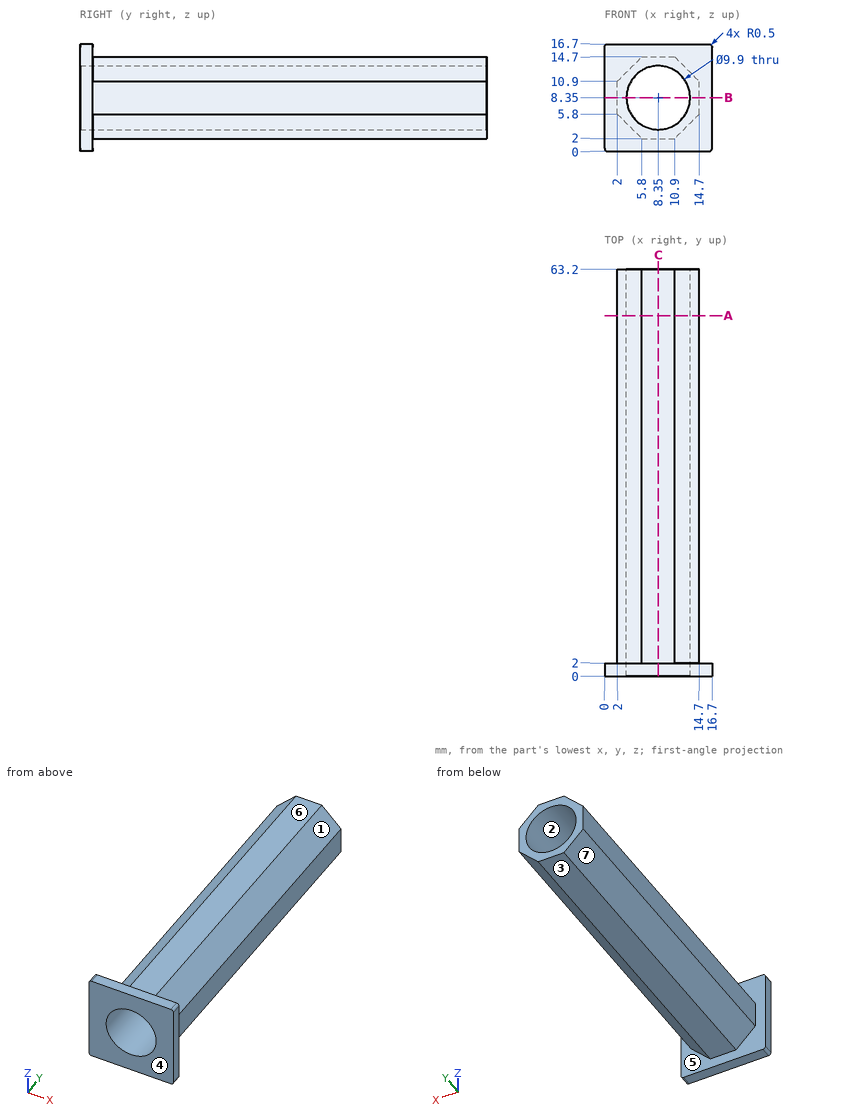
Verification items for this drawing (mm, ordinates from the low corner). A direction names the side the tool comes from. Coordinates: 2 decimals unless noted, no trailing zeros. Loops run counter-clockwise (first coordinate to the right, second up) from the corner with the lowest first, then second, coordinate; pieces in that order, holes last. Notation, with made-up numbers: (82, 11.5) - (108, 11.5) arc R20 cw to (108, 41.5) - close; hole circle Ø10 at (-20, 54.5). An arc over 180 degrees is marked (long way). One line per item, written item: value. Start each with the question number.
(1) Tool access check on the marked faces 4, 5, 6 and 7. Record the directions out of +Z, -Z, +X, -X, +Y, -Y that give a thin tool (end or side, any length) a straight path to the whole face; none if there is none.
(2) Mould release check, pull along X, two halves, no side actions. Record for the marked faces 1, 2 and 3: released by +X, released by -X, zero draft, split by the parting line, or undercut.
(3) Cross-section at C-C on x = 8.35. Enter the section's corners in (y, z), plus the area to 3 significant figures.
(4) Depth check by flat-ended pin: P1, Ø5.5, axis at x = 8, y = 34, coming from the +Z side; P2, Ø3, axis at x = 12.5, y = 12, coming from the -Z side; P3, Ø1.5, axis at y = 31, z = 9, coming from the -X side. Enter the tip coordinate at first touch or a pass-through.
(5) Cross-section at A-A on y = 56. Enter the section's corners in (x, z).
(6) Cross-section at B-B on z = 8.35. Enter the section's corners in (x, y).
(7) Material ranges on line 1 (Z direction, x = 8.35, y = 30); line 2 (Y direction, x = 3.5, z = 1.5); line 3 (Z direction, x = 10.25, y = 38), recorded low to high. Write a range as [from, to].
Results below:
1. face 4: +Z, -Z, +X, -X, -Y
1. face 5: +Y
1. face 6: +Z, +X, -X, +Y
1. face 7: -Z, -X, +Y
2. face 1: released by +X
2. face 2: undercut
2. face 3: zero draft
3. outline: (0, 0) - (2, 0) - (2, 2) - (63.2, 2) - (63.2, 3.4) - (0, 3.4) - close; (0, 13.3) - (63.2, 13.3) - (63.2, 14.7) - (2, 14.7) - (2, 16.7) - (0, 16.7) - close
3. area: 185 mm2
4. P1: stops at z = 14.7
4. P2: stops at z = 2.1
4. P3: stops at x = 2
5. outline: (2, 5.8) - (5.8, 2) - (10.9, 2) - (14.7, 5.8) - (14.7, 10.9) - (10.9, 14.7) - (5.8, 14.7) - (2, 10.9) - close; hole circle Ø9.9 at (8.35, 8.35)
6. outline: (0, 0) - (3.4, 0) - (3.4, 63.2) - (2, 63.2) - (2, 2) - (0, 2) - close; (13.3, 0) - (16.7, 0) - (16.7, 2) - (14.7, 2) - (14.7, 63.2) - (13.3, 63.2) - close
7. line 1: z = [2, 3.4], [13.3, 14.7]
7. line 2: y = [0, 2]
7. line 3: z = [2, 3.78], [12.92, 14.7]
